from build123d import *

# Parameters (mm, degrees)
BOSS_EXTRUDE1_DEPTH = 3


with BuildPart() as part:
    # Sketch2 → Boss-Extrude1 (new body)
    with BuildSketch(Plane(origin=(0, 0, 0), x_dir=(1, 0, 0), z_dir=(0, 1, 0))):
        Polygon((100, 288.675134595), (-100, 288.675134595), (-300, -57.735026919), (-250, -144.337567297), (200, 115.470053838), align=None)
        Polygon((300, -57.735026919), (200, 115.470053838), (-250, -144.337567297), (-200, -230.940107676), (200, -230.940107676), align=None)
    extrude(amount=BOSS_EXTRUDE1_DEPTH)


solid = part.part
Work out the finished part from the listing and answer in its coordinate system (mm). Coordinates: 2 decimals unless noted, no trailing zeros. Write each loop counter-clockwise with the first axis right and the second up, starting at its lowest first coordinate (ties: lowest second). Pieces come first, ordered by that corner, then holes. Notation, with made-up numbers: M 5,77.25 L 58,77.25 A27 cw 58,101.25 Z; hole C 63.5,58.5 d11. An arc over 180 degrees is marked long. Use one line per item in the form item = value. Start each with the question number.
1. The part is cut by section C-C (x = 130.5). Give the vertices of the cut face in (y, z), plus the area to 3 significant figures.
2. Straight lines are drawn through the part: probe 1 along X at (y, z) = (1.25, 106); probe 2 along X at (y, z) = (2.8, -0.5); probe 3 along Z at (x, y) = (-242, 1.65). For each, find the intervals that lie inside material, in ascending order. Write a range as from..to.
3. This flat-tipped pin is pushed along its axis until it touches: P1, Ø1.5, axis at y = 1, z = 96.5, coming from the +X side. Where does it stop, or does it pass through?
4. The part is cut by section A-A (y = 1.45). Give the vertices of the cut face in (x, z).
5. The part is cut by section B-B (z = 166.5). Give the vertices of the cut face in (x, y).
Evaluation:
q1.outline = M 0,-235.85 L 3,-235.85 L 3,230.94 L 0,230.94 Z
q1.area = 1,400 mm^2
q2.probe_1 = -272.13..272.13
q2.probe_2 = -266.38..266.38
q2.probe_3 = -42.72..158.19
q3.P1 = 278.05
q4.outline = M -300,57.74 L -100,-288.68 L 100,-288.68 L 300,57.74 L 200,230.94 L -200,230.94 Z
q5.outline = M -237.2,0 L 237.2,0 L 237.2,3 L -237.2,3 Z
